```python
from build123d import *

# Parameters (mm, degrees)
SKIZZE1_W                        = 275
SKIZZE1_H                        = 150
AUFSATZ_LINEAR_AUSTRAGEN1_DEPTH  = 3
SKIZZE2_W                        = 3
SKIZZE2_H                        = 144
SKIZZE2_W_2                      = 269
SKIZZE2_H_2                      = 3
AUFSATZ_LINEAR_AUSTRAGEN2_DEPTH  = 62
SKIZZE3_R                        = 4
AUFSATZ_LINEAR_AUSTRAGEN3_DEPTH  = 55
SKIZZE4_R                        = 1.55
SCHNITT_LINEAR_AUSTRAGEN1_DEPTH  = 168.018711527
SKIZZE9_R                        = 1.65
SCHNITT_LINEAR_AUSTRAGEN2_DEPTH  = 169.449547343
SKIZZE8_R                        = 2.2
SCHNITT_LINEAR_AUSTRAGEN3_DEPTH  = 10
SKIZZE10_R                       = 1.65
SCHNITT_LINEAR_AUSTRAGEN4_DEPTH  = 10
SKIZZE12_R                       = 2.15
SCHNITT_LINEAR_AUSTRAGEN5_DEPTH  = 10
SKIZZE13_W                       = 50
SKIZZE13_H                       = 5
SCHNITT_LINEAR_AUSTRAGEN6_DEPTH  = 3
SKIZZE14_W                       = 14
SKIZZE14_H                       = 8
SCHNITT_LINEAR_AUSTRAGEN7_DEPTH  = 3
SKIZZE20_R                       = 1.65
SCHNITT_LINEAR_AUSTRAGEN8_DEPTH  = 3
SKIZZE21_R                       = 1.65
SCHNITT_LINEAR_AUSTRAGEN9_DEPTH  = 3
SCHNITT_LINEAR_START             = -3
SKIZZE22_R                       = 1.65
SCHNITT_LINEAR_AUSTRAGEN10_DEPTH = 3
SKIZZE23_R                       = 1.65
SCHNITT_LINEAR_AUSTRAGEN11_DEPTH = 3
SKIZZE24_R                       = 1.65
SCHNITT_LINEAR_AUSTRAGEN12_DEPTH = 3


with BuildPart() as part:
    # Skizze1 → Aufsatz-Linear austragen1 (new body)
    with BuildSketch(Plane(origin=(0, 0, 0), x_dir=(1, 0, 0), z_dir=(0, 1, 0))):
        Rectangle(SKIZZE1_W, SKIZZE1_H)
    extrude(amount=AUFSATZ_LINEAR_AUSTRAGEN1_DEPTH)

    # Skizze2 → Aufsatz-Linear austragen2 (add)
    with BuildSketch(Plane(origin=(0, 3, 0), x_dir=(1, 0, 0), z_dir=(0, 1, 0))):
        with Locations((-136, 0)):
            Rectangle(SKIZZE2_W, SKIZZE2_H)
        with Locations((0, 73.5)):
            Rectangle(SKIZZE2_W_2, SKIZZE2_H_2)
        with Locations((-136, 73.5)):
            Rectangle(SKIZZE2_W, SKIZZE2_H_2)
        with Locations((136, 0)):
            Rectangle(SKIZZE2_W, SKIZZE2_H)
        with Locations((136, 73.5)):
            Rectangle(SKIZZE2_W, SKIZZE2_H_2)
        with Locations((0, -73.5)):
            Rectangle(SKIZZE2_W_2, SKIZZE2_H_2)
        with Locations((136, -73.5)):
            Rectangle(SKIZZE2_W, SKIZZE2_H_2)
        with Locations((-136, -73.5)):
            Rectangle(SKIZZE2_W, SKIZZE2_H_2)
    extrude(amount=AUFSATZ_LINEAR_AUSTRAGEN2_DEPTH)

    # Skizze3 → Aufsatz-Linear austragen3 (add)
    with BuildSketch(Plane(origin=(0, 3, 0), x_dir=(1, 0, 0), z_dir=(0, 1, 0))):
        with Locations(Location((-85.5, -66.5, 0), (0, 0, 90))):
            Circle(SKIZZE3_R)
        with Locations(Location((85.5, -66.5, 0), (0, 0, 90))):
            Circle(SKIZZE3_R)
    extrude(amount=AUFSATZ_LINEAR_AUSTRAGEN3_DEPTH)

    # Skizze4 → Schnitt-Linear austragen1 (cut, through all)
    with BuildSketch(Plane(origin=(0, 58, 0), x_dir=(1, 0, 0), z_dir=(0, 1, 0))):
        with Locations(Location((-85.5, -66.5, 0), (0, 0, 270))):
            Circle(SKIZZE4_R)
        with Locations(Location((85.5, -66.5, 0), (0, 0, 270))):
            Circle(SKIZZE4_R)
    extrude(amount=-SCHNITT_LINEAR_AUSTRAGEN1_DEPTH, mode=Mode.SUBTRACT)

    # Skizze9 → Schnitt-Linear austragen2 (cut, through all)
    with BuildSketch(Plane(origin=(0, 3, 0), x_dir=(1, 0, 0), z_dir=(0, 1, 0))):
        with Locations(Location((85.625, -4, 0), (0, 0, 270))):
            Circle(SKIZZE9_R)
    extrude(amount=-SCHNITT_LINEAR_AUSTRAGEN2_DEPTH, mode=Mode.SUBTRACT)

    # Skizze8 → Schnitt-Linear austragen3 (cut)
    with BuildSketch(Plane(origin=(0, 3, 0), x_dir=(1, 0, 0), z_dir=(0, 1, 0))):
        with Locations(Location((121.5, 15, 0), (0, 0, 270))):
            Circle(SKIZZE8_R)
        with Locations(Location((-121, 14.5, 0), (0, 0, 270))):
            Circle(SKIZZE8_R)
        with Locations(Location((-59.042286835, -1.5, 0), (0, 0, 270))):
            Circle(SKIZZE8_R)
        with Locations(Location((-114.042286835, -2.5, 0), (0, 0, 270))):
            Circle(SKIZZE8_R)
        with Locations(Location((-113.5, -27.5, 0), (0, 0, 270))):
            Circle(SKIZZE8_R)
    extrude(amount=-SCHNITT_LINEAR_AUSTRAGEN3_DEPTH, mode=Mode.SUBTRACT)

    # Skizze10 → Schnitt-Linear austragen4 (cut)
    with BuildSketch(Plane(origin=(0, 3, 0), x_dir=(1, 0, 0), z_dir=(0, 1, 0))):
        with Locations(Location((-129.5, 67, 0), (0, 0, 270))):
            Circle(SKIZZE10_R)
        with Locations(Location((129.5, 67, 0), (0, 0, 270))):
            Circle(SKIZZE10_R)
        with Locations(Location((129.5, -67, 0), (0, 0, 270))):
            Circle(SKIZZE10_R)
        with Locations(Location((-129.5, -67, 0), (0, 0, 270))):
            Circle(SKIZZE10_R)
    extrude(amount=-SCHNITT_LINEAR_AUSTRAGEN4_DEPTH, mode=Mode.SUBTRACT)

    # Skizze12 → Schnitt-Linear austragen5 (cut)
    with BuildSketch(Plane(origin=(137.5, 0, 0), x_dir=(0, 0, -1), z_dir=(1, 0, 0))):
        with BuildLine():
            ThreePointArc((-40.238883175, 43.36778368), (-48.991660734, 38.531578038), (-54.309023109, 30.062477887))
            Line((-54.309023109, 30.062477887), (-40.238883175, 43.36778368))
        make_face()
        with BuildLine():
            ThreePointArc((-55.182247429, 22.355155802), (-54.733751685, 19.485199861), (-53.874256158, 16.710481321))
            Line((-53.874256158, 16.710481321), (-26.931989392, 42.188202207))
            ThreePointArc((-26.931989392, 42.188202207), (-29.654390681, 43.201280071), (-32.494828488, 43.809316746))
            Line((-32.494828488, 43.809316746), (-55.182247429, 22.355155802))
        make_face()
        with BuildLine():
            Line((-22.550104474, 39.450328593), (-51.385310709, 12.182565916))
            ThreePointArc((-51.385310709, 12.182565916), (-49.78291784, 10.259756223), (-47.952908231, 8.552148289))
            Line((-47.952908231, 8.552148289), (-19.116994099, 35.820580383))
            ThreePointArc((-19.116994099, 35.820580383), (-20.719761902, 37.743077559), (-22.550104474, 39.450328593))
        make_face()
        with BuildLine():
            Line((-16.627265595, 31.293405466), (-43.571806367, 5.813534186))
            ThreePointArc((-43.571806367, 5.813534186), (-40.851994747, 4.800581914), (-38.014212853, 4.191942869))
            Line((-38.014212853, 4.191942869), (-15.318505409, 25.653941765))
            ThreePointArc((-15.318505409, 25.653941765), (-15.767750872, 28.521279567), (-16.627265595, 31.293405466))
        make_face()
        with BuildLine():
            Line((-16.186522357, 17.951543986), (-30.275365538, 4.628551629))
            ThreePointArc((-30.275365538, 4.628551629), (-21.508339266, 9.468421962), (-16.186522357, 17.951543986))
        make_face()
        with Locations((-51.25, 40)):
            Circle(SKIZZE12_R)
        with BuildLine():
            ThreePointArc((-19.760186439, 42.088590385), (-20.727228529, 41.562144639), (-21.306846696, 40.626004528))
            Line((-21.306846696, 40.626004528), (-19.760186439, 42.088590385))
        make_face()
        with BuildLine():
            Line((-19.760186439, 42.088590385), (-21.306846696, 40.626004528))
            ThreePointArc((-21.306846696, 40.626004528), (-19.566448735, 37.873415838), (-17.1, 40))
            ThreePointArc((-17.1, 40), (-17.922295372, 41.691064878), (-19.760186439, 42.088590385))
        make_face()
        with Locations((-19.25, 8)):
            Circle(SKIZZE12_R)
        with BuildLine():
            ThreePointArc((-50.747386311, 5.909574331), (-49.772771471, 6.437855361), (-49.190898067, 7.381453938))
            Line((-49.190898067, 7.381453938), (-50.747386311, 5.909574331))
        make_face()
        with BuildLine():
            Line((-50.747386311, 5.909574331), (-49.190898067, 7.381453938))
            ThreePointArc((-49.190898067, 7.381453938), (-49.122845897, 7.687405338), (-49.1, 8))
            ThreePointArc((-49.1, 8), (-52.938656186, 9.330766803), (-50.747386311, 5.909574331))
        make_face()
    extrude(amount=-SCHNITT_LINEAR_AUSTRAGEN5_DEPTH, mode=Mode.SUBTRACT)

    # Skizze13 → Schnitt-Linear austragen6 (cut)
    with BuildSketch(Plane.ZY.offset(137.5)):
        with Locations((35, 8.5)):
            Rectangle(SKIZZE13_W, SKIZZE13_H)
    extrude(amount=-SCHNITT_LINEAR_AUSTRAGEN6_DEPTH, mode=Mode.SUBTRACT)

    # Skizze14 → Schnitt-Linear austragen7 (cut)
    with BuildSketch(Plane.XY.offset(75)):
        with Locations((-32.525, 56.6)):
            Rectangle(SKIZZE14_W, SKIZZE14_H)
        with Locations((36.825, 56.6)):
            Rectangle(SKIZZE14_W, SKIZZE14_H)
    extrude(amount=-SCHNITT_LINEAR_AUSTRAGEN7_DEPTH, mode=Mode.SUBTRACT)

    # Skizze20 → Schnitt-Linear austragen8 (cut)
    with BuildSketch(Plane(origin=(0, 3, 0), x_dir=(1, 0, 0), z_dir=(0, 1, 0))):
        with Locations(Location((0, -41.062589667, 0), (0, 0, 270))):
            Circle(SKIZZE20_R)
        with Locations(Location((20, -41.062589667, 0), (0, 0, 270))):
            Circle(SKIZZE20_R)
    extrude(amount=-SCHNITT_LINEAR_AUSTRAGEN8_DEPTH, mode=Mode.SUBTRACT)

    # Skizze21 → Schnitt-Linear austragen9 (cut)
    with BuildSketch(Plane(origin=(137.5, 0, 0), x_dir=(0, 0, -1), z_dir=(1, 0, 0))):
        with Locations((-67, 52)):
            Circle(SKIZZE21_R)
        with Locations((-67, 13)):
            Circle(SKIZZE21_R)
        with Locations((67, 13)):
            Circle(SKIZZE21_R)
        with Locations((67, 52)):
            Circle(SKIZZE21_R)
    extrude(amount=-SCHNITT_LINEAR_AUSTRAGEN9_DEPTH, mode=Mode.SUBTRACT)

    # Skizze22 → Schnitt-Linear austragen10 (cut)
    with BuildSketch(Plane.ZY.offset(137.5).offset(SCHNITT_LINEAR_START)):
        with Locations(Location((-67, 52, 0), (0, 0, 180))):
            Circle(SKIZZE22_R)
        with Locations(Location((-67, 13, 0), (0, 0, 180))):
            Circle(SKIZZE22_R)
        with Locations(Location((67, 13, 0), (0, 0, 180))):
            Circle(SKIZZE22_R)
        with Locations(Location((67, 52, 0), (0, 0, 180))):
            Circle(SKIZZE22_R)
    extrude(amount=SCHNITT_LINEAR_AUSTRAGEN10_DEPTH, mode=Mode.SUBTRACT)

    # Skizze23 → Schnitt-Linear austragen11 (cut)
    with BuildSketch(Plane.XY.offset(75)):
        with Locations((-129.495008006, 43)):
            Circle(SKIZZE23_R)
        with Locations((-129.5, 22)):
            Circle(SKIZZE23_R)
        with Locations((129.5, 43)):
            Circle(SKIZZE23_R)
        with Locations((129.5, 22)):
            Circle(SKIZZE23_R)
    extrude(amount=-SCHNITT_LINEAR_AUSTRAGEN11_DEPTH, mode=Mode.SUBTRACT)

    # Skizze24 → Schnitt-Linear austragen12 (cut)
    with BuildSketch(Plane(origin=(0, 0, -75), x_dir=(-1, 0, 0), z_dir=(0, 0, -1)).offset(SCHNITT_LINEAR_START)):
        with Locations(Location((-129.5, 43, 0), (0, 0, 180))):
            Circle(SKIZZE24_R)
        with Locations(Location((-129.5, 22, 0), (0, 0, 180))):
            Circle(SKIZZE24_R)
        with Locations((129.5, 43)):
            Circle(SKIZZE24_R)
        with Locations(Location((129.5, 22, 0), (0, 0, 180))):
            Circle(SKIZZE24_R)
    extrude(amount=SCHNITT_LINEAR_AUSTRAGEN12_DEPTH, mode=Mode.SUBTRACT)


solid = part.part
```
Could you check a few things on this model? Use its own coordinates, in mm. A direction names the side the tool comes from. Give positions to 0.01 mm unless a question says otherwise; leave off trailing zeros. Write each loop counter-clockwise with the first axis right and the second up, starting at its lowest first coordinate (ties: lowest second). Pieces come first, ordered by that corner, then holes. Notation, with made-up numbers: (54, 86) -> (85, 86) arc R20 cw to (85, 108) -> close; hole circle Ø4 at (-13.5, 50). An arc over 180 degrees is marked (long way). Write each question's results on one line, items separated by ' | '.
1. I want a section at A-A, the plane z = -61. Write out the boundary of the cut face in (x, y).
Check sheet entries:
outline: (-137.5, 0) -> (137.5, 0) -> (137.5, 65) -> (134.5, 65) -> (134.5, 3) -> (-134.5, 3) -> (-134.5, 65) -> (-137.5, 65) -> close
2. I need wall thicknesses on L1, parallel to Z at x = -135.55, y = 52; L2, parallel to Y at x = -129.5, z = 73.15; L3, parallel to Z at x = 110, y = 27. Which ranges of each line are inside material? Lowest first, please.
Check sheet entries:
L1: z = -75 to -68.65, -65.35 to 65.35, 68.65 to 75 | L2: y = 0 to 20.35, 23.65 to 41.35, 44.65 to 65 | L3: z = -75 to -72, 72 to 75
3. On a 3-axis mill with a long thin cutter (end or side, diameter ignored), from which of +Z, -Z, +X, -X, +Y, -Y can I reach the whole of each face in a straight line? I mean faces 1 (the flat face through (-1, 65, -73)), 2 (the flat face through (136.02, 18.73, 29.91)), 3 (the flat face through (134.5, 34, 1)). Say none if no direction works.
Check sheet entries:
face 1: +Z, -Z, +X, -X, +Y | face 2: +X | face 3: +Y
4. If we mould it in two halves opening along Z, with no side actions, what happens to faces 4 (the flat face through (-2, 32, 75)), 5 (the flat face through (137.5, 32, 1)), 6 (the flat face through (-134.5, 34, 1))? For each: released by +Z, released by -Z, zero draft, split by the parting line, or undercut.
Check sheet entries:
face 4: released by +Z | face 5: zero draft | face 6: undercut
5. Will these pins go through, and if not, where does the flat tip stop? pin 1 Ø5.5 at (y, z) = (8, 51.25) entering from -X; pin 2 Ø2 at (x, z) = (39.5, 1) entering from +Y.
Check sheet entries:
pin 1: stops at x = -137.5 | pin 2: stops at y = 3
6. I want a section at B-B, the plane x = 108. Write out the boundary of the cut face in (y, z), then the cut area to 3 significant figures.
Check sheet entries:
outline: (0, -75) -> (65, -75) -> (65, -72) -> (3, -72) -> (3, 72) -> (65, 72) -> (65, 75) -> (0, 75) -> close | area: 822 mm²
